Design review of the part built by this model. Coordinates are the model's own, in mm. Face numbers are marked on the shaded views. A direction names the side the tool comes from. Give positions to 0.01 mm unless a question says otherwise; leave off trailing zeros. Loops run counter-clockwise (first coordinate to the right, second up) from the corner with the lowest first, then second, coordinate; pieces in that order, holes last. Notation, with made-up numbers: (45.5, -5.5) - (95.5, -5.5) arc R33 ccw to (95.5, 30.5) - close; hole circle Ø2 at (53.25, 4.25). An arc over 180 degrees is marked (long way). Write each question's results on one line, items separated by ' | '.
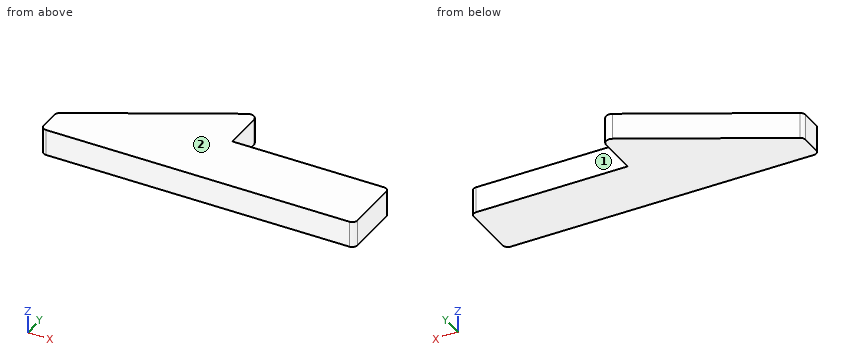
from build123d import *

# Parameters (mm, degrees)
F1_DEPTH = 6.35


with BuildPart() as f1:
    # F0 (on Top) → F1 (new body)
    with BuildSketch(Plane.XY):
        with BuildLine():
            ThreePointArc((52.952157, 17.634291), (52.580183, 18.532317), (51.682157, 18.904291))
            Line((51.682157, 18.904291), (14.852157, 18.904291))
            Line((14.852157, 18.904291), (14.852157, 28.413579))
            ThreePointArc((14.852157, 28.413579), (14.0717, 29.787865), (12.491624, 29.821603))
            Line((12.491624, 29.821603), (-22.581282, 10.882234))
            ThreePointArc((-22.581282, 10.882234), (-23.068546, 10.415343), (-23.247843, 9.764754))
            Line((-23.247843, 9.764754), (-23.247843, 4.934291))
            ThreePointArc((-23.247843, 4.934291), (-22.875868, 4.036266), (-21.977843, 3.664291))
            Line((-21.977843, 3.664291), (51.682157, 3.664291))
            ThreePointArc((51.682157, 3.664291), (52.580183, 4.036266), (52.952157, 4.934291))
            Line((52.952157, 4.934291), (52.952157, 17.634291))
        make_face()
    extrude(amount=F1_DEPTH)


solid = f1.part
(1) Take a section at A-A on z = 2. Give the boundary of the cut face in (x, y).
Answers below:
outline: (-23.25, 4.93) arc R1.27 ccw to (-21.98, 3.66) - (51.68, 3.66) arc R1.27 ccw to (52.95, 4.93) - (52.95, 17.63) arc R1.27 ccw to (51.68, 18.9) - (14.85, 18.9) - (14.85, 28.41) arc R1.6 ccw to (12.49, 29.82) - (-22.58, 10.88) arc R1.27 ccw to (-23.25, 9.76) - close
(2) Take a section at B-B on x = 36.5. Give the boundary of the cut face in (y, z).
Answers below:
outline: (3.66, 0) - (18.9, 0) - (18.9, 6.35) - (3.66, 6.35) - close
(3) Insertion check: P1, Ø1, axis at x = 18, z = 3.5, coming from the +Y side; P2, Ø3, axis at y = 24.5, z = 5, coming from the -X side. Each pin has a flat end and moves straight along its axis. Give the tip position at first contact, or say it passes through.
Answers below:
P1: y = 18.9 | P2: x = -0.14
(4) Take a section at C-C on y = 26. Give the boundary of the cut face in (x, z), plus the area to 3 significant figures.
Answers below:
outline: (5.41, 0) - (14.85, 0) - (14.85, 6.35) - (5.41, 6.35) - close | area: 59.9 mm2
(5) Wall thickness on line 1 along Y through (x, z) = (29, 4.5); line 2 along X through (y, z) = (20.75, 1.75); line 3 along X through (y, z) = (18.25, 0.75): over which ranges is each line inside the solid? List them lowest first. Write a range as from..to.
Answers below:
line 1: 3.66..18.9 | line 2: -4.31..14.85 | line 3: -8.94..52.79
(6) Tool access review of the marked faces 1 and 2: name each direction out of +Z, -Z, +X, -X, +Y, -Y from which nothing blocks a thin tool from reaching the whole face with its end or side.
Answers below:
face 1: +Z, -Z, +X, +Y | face 2: +Z, +X, -X, +Y, -Y
